Source: CAD feature listing. Evaluate the final solid. Frame: model axes, mm. Face numbers are marked on the shaded views. Give positions to 0.01 mm unless a question says otherwise; leave off trailing zeros. Loops run counter-clockwise (first coordinate to the right, second up) from the corner with the lowest first, then second, coordinate; pieces in that order, holes last.
```python
from build123d import *

# Parameters (mm, degrees)
CYLINDER1331_R                     = 1.6
CYLINDER1331_DEPTH                 = 60
CYLINDER1332_R                     = 1.6
CYLINDER1332_DEPTH                 = 60
CYLINDER1333_R                     = 1.6
CYLINDER1333_DEPTH                 = 60
CYLINDER1330_R                     = 1.6
CYLINDER1330_DEPTH                 = 60
FUSION248002050200_PLACEMENT_ANGLE = 90
CYLINDER1329_R                     = 2.7
CYLINDER1329_DEPTH                 = 15
CYLINDER1328_R                     = 2.7
CYLINDER1328_DEPTH                 = 15
CYLINDER1327_R                     = 4.75
CYLINDER1327_DEPTH                 = 27
CYLINDER1326_R                     = 5.2
CYLINDER1326_DEPTH                 = 9.5
CYLINDER1323_R                     = 14.1
CYLINDER1323_DEPTH                 = 5
CYLINDER1324_R                     = 14.1
CYLINDER1324_DEPTH                 = 5
CYLINDER1325_R                     = 5.2
CYLINDER1325_DEPTH                 = 9.5
FUSION248002050201_PLACEMENT_ANGLE = 90
BOX545_W                           = 32
BOX545_H                           = 66
BOX545_DEPTH                       = 10


with BuildPart() as cylinder1331:
    # Cylinder1331 → Cylinder1331 (new body)
    with BuildSketch(Plane(origin=(432, 67, 100), x_dir=(0, 0, -1), z_dir=(1, 0, 0))):
        Circle(CYLINDER1331_R)
    extrude(amount=CYLINDER1331_DEPTH)


with BuildPart() as cylinder1332:
    # Cylinder1332 → Cylinder1332 (new body)
    with BuildSketch(Plane(origin=(432, 93.5, 94), x_dir=(0, 0, -1), z_dir=(1, 0, 0))):
        Circle(CYLINDER1332_R)
    extrude(amount=CYLINDER1332_DEPTH)


with BuildPart() as cylinder1333:
    # Cylinder1333 → Cylinder1333 (new body)
    with BuildSketch(Plane(origin=(432, 76.5, 94), x_dir=(0, 0, -1), z_dir=(1, 0, 0))):
        Circle(CYLINDER1333_R)
    extrude(amount=CYLINDER1333_DEPTH)


with BuildPart() as fusion248002050200:
    # Cylinder1330 → Cylinder1330 (new body)
    with BuildSketch(Plane(origin=(432, 103, 100), x_dir=(0, 0, -1), z_dir=(1, 0, 0))):
        Circle(CYLINDER1330_R)
    extrude(amount=CYLINDER1330_DEPTH)

    # Fusion248002050200: union Cylinder1331, Cylinder1332, Cylinder1333
    add(cylinder1331.part)
    add(cylinder1332.part)
    add(cylinder1333.part)


with BuildPart() as fusion248002050200_1:
    # Fusion248002050200 placement: moved
    add(fusion248002050200.part.moved(Location((-82, -50, 452))).rotate(Axis((-82, -50, 452), (0, 1, 0)), FUSION248002050200_PLACEMENT_ANGLE))


with BuildPart() as cylinder1329:
    # Cylinder1329 → Cylinder1329 (new body)
    with BuildSketch(Plane(origin=(428.75, 103, 100), x_dir=(0, 0, -1), z_dir=(1, 0, 0))):
        Circle(CYLINDER1329_R)
    extrude(amount=CYLINDER1329_DEPTH)


with BuildPart() as cylinder1328:
    # Cylinder1328 → Cylinder1328 (new body)
    with BuildSketch(Plane(origin=(428.75, 67, 100), x_dir=(0, 0, -1), z_dir=(1, 0, 0))):
        Circle(CYLINDER1328_R)
    extrude(amount=CYLINDER1328_DEPTH)


with BuildPart() as cylinder1327:
    # Cylinder1327 → Cylinder1327 (new body)
    with BuildSketch(Plane(origin=(441.5, 85, 87), x_dir=(1, 0, 0), z_dir=(0, 0, 1))):
        Circle(CYLINDER1327_R)
    extrude(amount=CYLINDER1327_DEPTH)


with BuildPart() as cylinder1326:
    # Cylinder1326 → Cylinder1326 (new body)
    with BuildSketch(Plane(origin=(434.75, 102.5, 100), x_dir=(0, 0, -1), z_dir=(1, 0, 0))):
        Circle(CYLINDER1326_R)
    extrude(amount=CYLINDER1326_DEPTH)


with BuildPart() as fusion248002050199:
    # Cylinder1323 → Cylinder1323 (new body)
    with BuildSketch(Plane(origin=(437, 102.5, 100), x_dir=(0, 0, -1), z_dir=(1, 0, 0))):
        Circle(CYLINDER1323_R)
    extrude(amount=CYLINDER1323_DEPTH)

    # Fusion248002050199: union Cylinder1326
    add(cylinder1326.part)


with BuildPart() as fusion248002050199_1:
    # Fusion248002050199 placement: moved
    add(fusion248002050199.part.moved(Location((2, 0.5, 0))))


with BuildPart() as cylinder1324:
    # Cylinder1324 → Cylinder1324 (new body)
    with BuildSketch(Plane(origin=(437, 67.5, 100), x_dir=(0, 0, -1), z_dir=(1, 0, 0))):
        Circle(CYLINDER1324_R)
    extrude(amount=CYLINDER1324_DEPTH)


with BuildPart() as fusion248002050201:
    # Cylinder1325 → Cylinder1325 (new body)
    with BuildSketch(Plane(origin=(434.75, 67.5, 100), x_dir=(0, 0, -1), z_dir=(1, 0, 0))):
        Circle(CYLINDER1325_R)
    extrude(amount=CYLINDER1325_DEPTH)

    # Fusion248002050198: union Cylinder1324
    add(cylinder1324.part)


with BuildPart() as fusion248002050201_1:
    # Fusion248002050198 placement: moved
    add(fusion248002050201.part.moved(Location((2, -0.5, 0))))

    # Fusion248002050201: union Cylinder1329, Cylinder1328, Cylinder1327, Fusion248002050199
    add(cylinder1329.part)
    add(cylinder1328.part)
    add(cylinder1327.part)
    add(fusion248002050199_1.part)


with BuildPart() as fusion248002050201_2:
    # Fusion248002050201 placement: moved
    add(fusion248002050201_1.part.moved(Location((118, -50, -432))).rotate(Axis((118, -50, -432), (0, -1, 0)), FUSION248002050201_PLACEMENT_ANGLE))


with BuildPart() as bucket_gears_holes:
    # Box545 → Box545 (new body)
    with BuildSketch(Plane(origin=(1.5, 2, 0), x_dir=(1, 0, 0), z_dir=(0, 0, 1))):
        with Locations((16, 33)):
            Rectangle(BOX545_W, BOX545_H)
    extrude(amount=BOX545_DEPTH)

    # Cut: cut Fusion248002050201
    add(fusion248002050201_2.part, mode=Mode.SUBTRACT)

    # Cut014344: cut Fusion248002050200
    add(fusion248002050200_1.part, mode=Mode.SUBTRACT)


solid = bucket_gears_holes.part
```
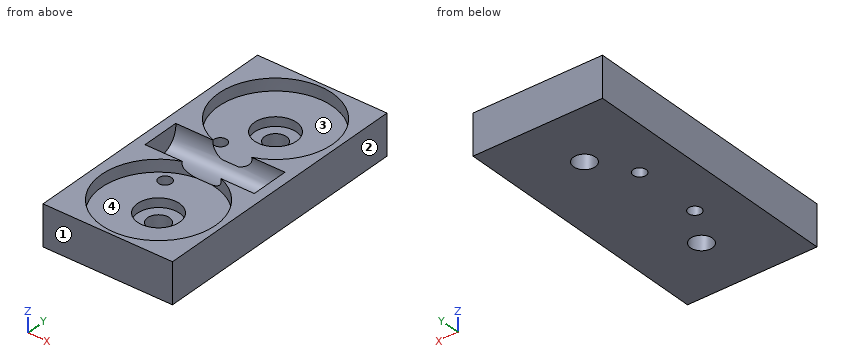
(1) Section A-A, the plane x = 18. Return the cut outline in (y, z), then the cut area to 3 significant figures.
A:
outline: (2, 0) - (14.3, 0) - (14.3, 4.75) - (11.8, 4.75) - (11.8, 7) - (2.9, 7) - (2.9, 10) - (2, 10) - close; (19.7, 0) - (50.3, 0) - (50.3, 4.75) - (47.8, 4.75) - (47.8, 7) - (39.04, 7) arc R4.75 cw to (30.96, 7) - (22.2, 7) - (22.2, 4.75) - (19.7, 4.75) - close; (55.7, 0) - (68, 0) - (68, 10) - (67.1, 10) - (67.1, 7) - (58.2, 7) - (58.2, 4.75) - (55.7, 4.75) - close
area: 356 mm2
(2) Section B-B, the plane y = 27.5. Return the cut outline in (x, z).
A:
outline: (1.5, 0) - (10.75, 0) - (10.75, 7) - (8.59, 7) - (8.59, 10) - (1.5, 10) - close; (13.25, 0) - (33.5, 0) - (33.5, 10) - (27.41, 10) - (27.41, 7) - (13.25, 7) - close
(3) First-contact query: pin 1 (4 mm diameter, centred on x = 12, y = 26.5, fed in from +Z); pin 2 (1 mm diameter, centred on x = 8, y = 34.5, fed in from +Z); pin 3 (3 mm diameter, centred on x = 18, y = 17, fed in from +Z). Flat tips, straight axial feed; report the tip coordinate or a pass-through.
A:
pin 1: stops at z = 7
pin 2: stops at z = 4.86
pin 3: passes through
(4) Mould query, pull axis X, two halves, no side actions, for the marked faces 1, 2, 3 and 4. Classes: pulls with the +X half, pulls with the -X half, needs draft (parallel to the pull), parting line crosses it, or undercut.
A:
face 1: needs draft
face 2: pulls with the +X half
face 3: undercut
face 4: undercut
(5) Ray query, line 1 along Y through (x, z) = (18, 2.4); line 2 along X through (y, z) = (53, 6.25); line 3 along X through (y, z) = (43.5, 5.25). Return the intervals inside material, ascending.
A:
line 1: y = 2 to 14.3, 19.7 to 50.3, 55.7 to 68
line 2: x = 1.5 to 12.8, 23.2 to 33.5
line 3: x = 1.5 to 10.4, 13.6 to 33.5
(6) Section C-C, the plane z = 6. Return the cut outline in (x, y).
A:
outline: (1.5, 2) - (33.5, 2) - (33.5, 68) - (1.5, 68) - close; hole (4, 31.79) - (31, 31.79) - (31, 38.21) - (4, 38.21) - close; hole circle Ø3.2 at (12, 26.5); hole circle Ø3.2 at (12, 43.5); hole circle Ø10.4 at (18, 17); hole circle Ø10.4 at (18, 53)
(7) Section D-D, the plane y = 35. Return the cut outline in (x, z).
A:
outline: (1.5, 0) - (33.5, 0) - (33.5, 10) - (31, 10) - (31, 4.75) - (4, 4.75) - (4, 10) - (1.5, 10) - close
